```python
from build123d import *

# Parameters (mm, degrees)
IZIM1_R                     = 0.95
IZIM1_R_2                   = 2.5
Y_KSEKLIK_EKSTR_ZYON4_DEPTH = 1.1
IZIM2_W                     = 15.9
IZIM2_H                     = 3.9
IZIM2_R                     = 0.95
Y_KSEKLIK_EKSTR_ZYON5_DEPTH = 3.9


with BuildPart() as part:
    # Çizim1 → Yükseklik-Ekstrüzyon4 (new body)
    with BuildSketch(Plane.XY):
        with BuildLine():
            ThreePointArc((-16, -8.354789046), (-10.092299035, -14.964892254), (-1.75, -17.964965906))
            Line((-1.75, -17.964965906), (-1.75, -16.464965906))
            Line((-1.75, -16.464965906), (1.75, -16.464965906))
            Line((1.75, -16.464965906), (1.75, -17.964965906))
            ThreePointArc((1.75, -17.964965906), (10.092299035, -14.964892254), (16, -8.354789046))
            Line((16, -8.354789046), (16, 8.354789046))
            ThreePointArc((16, 8.354789046), (10.092299035, 14.964892254), (1.75, 17.964965906))
            Line((1.75, 17.964965906), (1.75, 16.464965906))
            Line((1.75, 16.464965906), (-1.75, 16.464965906))
            Line((-1.75, 16.464965906), (-1.75, 17.964965906))
            ThreePointArc((-1.75, 17.964965906), (-10.092299035, 14.964892254), (-16, 8.354789046))
            Line((-16, 8.354789046), (-16, -8.354789046))
        make_face()
        with Locations((-6, -9.939079606)):
            Circle(IZIM1_R, mode=Mode.SUBTRACT)
        with Locations((-3, -9.939079606)):
            Circle(IZIM1_R, mode=Mode.SUBTRACT)
        with Locations((0, -9.939079606)):
            Circle(IZIM1_R, mode=Mode.SUBTRACT)
        with Locations((3, -9.939079606)):
            Circle(IZIM1_R, mode=Mode.SUBTRACT)
        with Locations((6, -9.939079606)):
            Circle(IZIM1_R, mode=Mode.SUBTRACT)
        with Locations((-9.5, 0)):
            Circle(IZIM1_R_2, mode=Mode.SUBTRACT)
        with Locations((9.5, 0)):
            Circle(IZIM1_R_2, mode=Mode.SUBTRACT)
    extrude(amount=Y_KSEKLIK_EKSTR_ZYON4_DEPTH)

    # Çizim2 → Yükseklik-Ekstrüzyon5 (add)
    with BuildSketch(Plane.XY.offset(1.1)):
        with Locations((0, -9.939079606)):
            Rectangle(IZIM2_W, IZIM2_H)
        with Locations((-6, -9.939079606)):
            Circle(IZIM2_R, mode=Mode.SUBTRACT)
        with Locations((3, -9.939079606)):
            Circle(IZIM2_R, mode=Mode.SUBTRACT)
        with Locations((0, -9.939079606)):
            Circle(IZIM2_R, mode=Mode.SUBTRACT)
        with Locations((6, -9.939079606)):
            Circle(IZIM2_R, mode=Mode.SUBTRACT)
        with Locations((-3, -9.939079606)):
            Circle(IZIM2_R, mode=Mode.SUBTRACT)
    extrude(amount=Y_KSEKLIK_EKSTR_ZYON5_DEPTH)


solid = part.part
```
The listing builds one solid part. Answer for the finished solid, in the listing's coordinates (mm). A direction names the side the tool comes from. Round coordinates to 2 decimals unless told otherwise and drop trailing zeros. Loops run counter-clockwise (first coordinate to the right, second up) from the corner with the lowest first, then second, coordinate; pieces in that order, holes last.
1) A cutting plane is placed at D-D on x = 9. Determine the outline of the cut face in (y, z), plus the area to 3 significant figures.
Outcome:
outline: (-15.65, 0) - (-2.45, 0) - (-2.45, 1.1) - (-15.65, 1.1) - close; (2.45, 0) - (15.65, 0) - (15.65, 1.1) - (2.45, 1.1) - close
area: 29.0 mm2
2) Given P1, Ø6, axis at x = -9.5, y = 0, coming from the -Z side; P2, Ø1.2, axis at y = -17, z = 0.5, coming from the +X side; P3, Ø3, axis at y = -12.5, z = 4.5, coming from the +X side; P4, Ø6, axis at x = 10, y = 8.5, coming from the +Z side, each flat-ended and moving along its own axis, determine where each tip first touches the part or whether it passes through.
Outcome:
P1: stops at z = 0
P2: stops at x = 7.54
P3: stops at x = 7.95
P4: stops at z = 1.1
3) For a pull along X with two mould halves and no side action, classify faces 1 (the face through (-0.1, -8.6, 5)), 2 (the face through (16, -0.1, 0.5)), 3 (the face through (0, 16.465, 0.5)) as released by +X, released by -X, zero draft, split by the parting line, or undercut.
Outcome:
face 1: zero draft
face 2: released by +X
face 3: undercut
4) Consider line 1 (Y direction, x = 3, z = 1.7); line 2 (Z direction, x = -2.5, y = -3); line 3 (X direction, y = -16, z = 0.65). Determine where each line is inside the solid, lowest interval first.
Outcome:
line 1: y = -11.89 to -10.89, -8.99 to -7.99
line 2: z = 0 to 1.1
line 3: x = -8.35 to 8.35
5) A cutting plane is placed at A-A on y = -2. Determine the outline of the cut face in (x, z), plus the area to 3 significant figures.
Outcome:
outline: (-16, 0) - (-11, 0) - (-11, 1.1) - (-16, 1.1) - close; (-8, 0) - (8, 0) - (8, 1.1) - (-8, 1.1) - close; (11, 0) - (16, 0) - (16, 1.1) - (11, 1.1) - close
area: 28.6 mm2
6) A cutting plane is placed at C-C on z = 2.5. Determine the outline of the cut face in (x, y), plus the area to 3 significant figures.
Outcome:
outline: (-7.95, -11.89) - (7.95, -11.89) - (7.95, -7.99) - (-7.95, -7.99) - close; hole circle Ø1.9 at (-6, -9.94); hole circle Ø1.9 at (-3, -9.94); hole circle Ø1.9 at (0, -9.94); hole circle Ø1.9 at (3, -9.94); hole circle Ø1.9 at (6, -9.94)
area: 47.8 mm2
7) For faces 4 (the face through (0, -11.889, 3)), 5 (the face through (0, -7.989, 3)), 6 (the face through (-7.95, -10, 3)), 7 (the face through (-1.75, -17.2, 0.5)), determine the directions among +Z, -Z, +X, -X, +Y, -Y from which every point of the face is accessible in a straight line to the end or side of a thin tool.
Outcome:
face 4: +Z, +X, -X, -Y
face 5: +Z, +X, -X, +Y
face 6: +Z, -X, +Y, -Y
face 7: +Z, -Z, -Y
8) A cutting plane is placed at B-B on x = 0. Determine the outline of the cut face in (y, z).
Outcome:
outline: (-16.46, 0) - (-10.89, 0) - (-10.89, 5) - (-11.89, 5) - (-11.89, 1.1) - (-16.46, 1.1) - close; (-8.99, 0) - (16.46, 0) - (16.46, 1.1) - (-7.99, 1.1) - (-7.99, 5) - (-8.99, 5) - close
